```python
from build123d import *

# Parameters (mm, degrees)
SKETCH_1_W          = 31
SKETCH_1_H          = 38
EXTRUDE_1_DEPTH     = 40.75
SKETCH_2_W          = 8
SKETCH_2_H          = 16.5
CUT_EXTRUDE_1_DEPTH = 40.75
SKETCH_3_W          = 25
SKETCH_3_H          = 34.75
CUT_EXTRUDE_2_DEPTH = 34.5
SKETCH_4_R          = 12.5
CUT_EXTRUDE_3_DEPTH = 34.5
SKETCH_5_R          = 1.6
EXTRUDE_2_DEPTH     = 3
SKETCH_6_W          = 31
SKETCH_6_H          = 16.5
CUT_EXTRUDE_4_DEPTH = 8
SKETCH_7_W          = 24
SKETCH_7_H          = 5
EXTRUDE_3_DEPTH     = 19.7
SKETCH_8_R          = 1.25
CUT_EXTRUDE_5_DEPTH = 20.7
FILLET_1_R          = 2


with BuildPart() as part:
    # 草图1 → 凸台-拉伸1 (new body)
    with BuildSketch(Plane.XY):
        with Locations((15.5, 19)):
            Rectangle(SKETCH_1_W, SKETCH_1_H)
    extrude(amount=-EXTRUDE_1_DEPTH)

    # 草图2 → 切除-拉伸1 (cut)
    with BuildSketch(Plane(origin=(31, 0, 0), x_dir=(0, 0, -1), z_dir=(1, 0, 0))):
        with Locations((36.75, 29.75)):
            Rectangle(SKETCH_2_W, SKETCH_2_H)
    extrude(amount=-CUT_EXTRUDE_1_DEPTH, mode=Mode.SUBTRACT)

    # 草图3 → 切除-拉伸2 (cut)
    with BuildSketch(Plane(origin=(0, 38, 0), x_dir=(1, 0, 0), z_dir=(0, 1, 0))):
        with Locations((15.5, 20.375)):
            Rectangle(SKETCH_3_W, SKETCH_3_H)
    extrude(amount=-CUT_EXTRUDE_2_DEPTH, mode=Mode.SUBTRACT)

    # 草图4 → 切除-拉伸3 (cut)
    with BuildSketch(Plane.XY):
        with Locations((15.5, 38)):
            Circle(SKETCH_4_R)
    extrude(amount=-CUT_EXTRUDE_3_DEPTH, mode=Mode.SUBTRACT)

    # 草图5 → 凸台-拉伸2 (add)
    with BuildSketch(Plane(origin=(0, 38, 0), x_dir=(1, 0, 0), z_dir=(0, 1, 0))):
        with BuildLine():
            Line((36, 23.375), (31, 23.375))
            Line((31, 23.375), (31, 17.375))
            Line((31, 17.375), (36, 17.375))
            ThreePointArc((36, 17.375), (39, 20.375), (36, 23.375))
        make_face()
        with Locations((36, 20.375)):
            Circle(SKETCH_5_R, mode=Mode.SUBTRACT)
        with BuildLine():
            Line((0, 23.375), (0, 17.375))
            Line((0, 17.375), (-5, 17.375))
            ThreePointArc((-5, 17.375), (-8, 20.375), (-5, 23.375))
            Line((-5, 23.375), (0, 23.375))
        make_face()
        with Locations((-5, 20.375)):
            Circle(SKETCH_5_R, mode=Mode.SUBTRACT)
    extrude(amount=-EXTRUDE_2_DEPTH)

    # 草图6 → 切除-拉伸4 (cut)
    with BuildSketch(Plane.XY):
        with Locations((15.5, 29.75)):
            Rectangle(SKETCH_6_W, SKETCH_6_H)
    extrude(amount=-CUT_EXTRUDE_4_DEPTH, mode=Mode.SUBTRACT)

    # 草图7 → 凸台-拉伸3 (add)
    with BuildSketch(Plane.XY):
        with Locations((15.5, 2.5)):
            Rectangle(SKETCH_7_W, SKETCH_7_H)
    extrude(amount=EXTRUDE_3_DEPTH)

    # 草图8 → 切除-拉伸5 (cut)
    with BuildSketch(Plane(origin=(0, 5, 0), x_dir=(1, 0, 0), z_dir=(0, 1, 0))):
        with Locations((6.5, -14.7)):
            Circle(SKETCH_8_R)
        with Locations((24.5, -14.7)):
            Circle(SKETCH_8_R)
    extrude(amount=-CUT_EXTRUDE_5_DEPTH, mode=Mode.SUBTRACT)

    # 圆角1
    fillet_1_edges = [part.edges().sort_by_distance(p)[0] for p in [
        (3.5, 2.5, 0),
        (27.5, 2.5, 0),
        (15.5, 5, 0),
    ]]
    fillet(fillet_1_edges, radius=FILLET_1_R)


solid = part.part
```
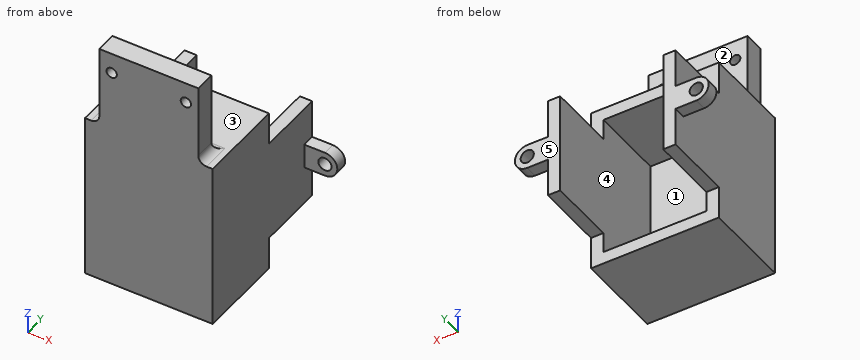
CAD build for the part. Positions are in the model's coordinates, mm. Face numbers are marked on the shaded views. A direction names the side the tool comes from. Round coordinates to 2 decimals unless told otherwise and drop trailing zeros. Order: outer loops, then holes, each group sorted by start corner. A loop starts at its lowest first (then second) coordinate and runs counter-clockwise, first axis right, second up.
Item 1: Mould opens along Z. For the marked faces 1, 2 and 3 say: pulls with the +Z half, pulls with the -Z half, needs draft (parallel to the pull), parting line crosses it, or undercut.
Item 2: Probe line 1 along Z through (x, y) = (20, 7.5); line 2 along Z through (x, y) = (6.5, 2.75); line 3 along X through (y, z) = (2.15, 14.7). List the from-to ranges inside material, lowest first.
Item 3: Saw through at B-B on z = 14.7. Write the cut outline in (x, y).
Item 4: Pin check, flat tips, straight feed: pin 1 (10.5 mm diameter, centred on y = 18.5, z = -15.5, fed in from +X); pin 2 (0.9 mm diameter, centred on x = 33.5, y = 36.5, fed in from +Z) (3 decimals); pin 3 (8 mm diameter, centred on y = 15, z = -12, fed in from -X). Stop position of each tip, or through.
Item 5: Saw through at A-A on y = 31.5. Write the cut outline in (x, z), then the cut area to 4 significant figures.
Item 6: Saw through at D-D on z = -10.5. Write the cut outline in (x, y), then the cut area to 4 significant figures.
Item 7: Saw through at C-C on x = 7. Write the cut outline in (y, z).
Item 8: Tool access for the marked faces 4 and 5: list every direction of +Z, -Z, +X, -X, +Y, -Y with a clear straight run to the whole face (end or side of a thin tool).
Reported:
1. face 1: undercut
1. face 2: needs draft
1. face 3: pulls with the +Z half
2. line 1: z = -40.75 to -37.75, -3 to 0
2. line 2: z = -40.75 to 13.45, 15.95 to 19.7
2. line 3: x = 3.5 to 5.25, 7.75 to 23.25, 25.75 to 27.5
3. outline: (3.5, 0) - (5.25, 0) - (5.25, 5) - (3.5, 5) - close; (7.75, 0) - (23.25, 0) - (23.25, 5) - (7.75, 5) - close; (25.75, 0) - (27.5, 0) - (27.5, 5) - (25.75, 5) - close
4. pin 1: stops at x = 31
4. pin 2: stops at z = -17.375
4. pin 3: stops at x = 0
5. outline: (0, -32.75) - (3, -32.75) - (3, -8) - (0, -8) - close; (28, -32.75) - (31, -32.75) - (31, -8) - (28, -8) - close
5. area: 148.5 mm2
6. outline: (0, 0) - (31, 0) - (31, 38) - (28, 38) - (28, 3.5) - (3, 3.5) - (3, 38) - (0, 38) - close
6. area: 315.5 mm2
7. outline: (0, -40.75) - (21.5, -40.75) - (21.5, -37.75) - (3.5, -37.75) - (3.5, -3) - (21.5, -3) - (21.5, 0) - (7, 0) arc R2 cw to (5, 2) - (5, 13.55) - (0, 13.55) - close; (0, 15.85) - (5, 15.85) - (5, 19.7) - (0, 19.7) - close
8. face 4: +Y
8. face 5: +Z, -Z, +X, -X, +Y
